The model under review builds one solid part; all positions refer to its coordinate system, in mm. Face numbers are marked on the shaded views. A direction names the side the tool comes from. Give positions to 0.01 mm unless a question says otherwise; leave off trailing zeros. Loops run counter-clockwise (first coordinate to the right, second up) from the corner with the lowest first, then second, coordinate; pieces in that order, holes last. Notation, with made-up numbers: M -29.5,-23.75 L 21.5,-23.75 A21 cw 21.5,4.25 Z; hole C 40.25,-38 d4. An arc over 180 degrees is marked long. Return JSON: item names as keys, results as strings.
```python
from build123d import *

# Parameters (mm, degrees)
BOSS_EXTRUDE1_DEPTH = 3
SKETCH2_R           = 3.8
BOSS_EXTRUDE2_DEPTH = 10
SKETCH3_R           = 1.7
CUT_EXTRUDE1_DEPTH  = 20
SKETCH5_R           = 1.1
SKETCH5_W           = 14
SKETCH5_H           = 24
CUT_EXTRUDE2_DEPTH  = 20
SKETCH6_W           = 3
SKETCH6_H           = 20
BOSS_EXTRUDE3_DEPTH = 50
FILLET2_START       = 7
FILLET2_DEPTH       = 2.5


with BuildPart() as part:
    # Sketch1 → Boss-Extrude1 (new body)
    with BuildSketch(Plane.XY):
        with BuildLine():
            Line((-9.5, 6.480740698), (-9.5, 66.480740698))
            Line((-9.5, 66.480740698), (9.5, 66.480740698))
            Line((9.5, 66.480740698), (9.5, 6.480740698))
            ThreePointArc((9.5, 6.480740698), (0, -11.5), (-9.5, 6.480740698))
        make_face()
    extrude(amount=BOSS_EXTRUDE1_DEPTH)

    # Sketch2 → Boss-Extrude2 (add)
    with BuildSketch(Plane.XY.offset(3)):
        Circle(SKETCH2_R)
    extrude(amount=BOSS_EXTRUDE2_DEPTH)

    # Sketch3 → Cut-Extrude1 (cut)
    with BuildSketch(Plane(origin=(0, 0, 0), x_dir=(-1, 0, 0), z_dir=(0, 0, -1))):
        Circle(SKETCH3_R)
    extrude(amount=-CUT_EXTRUDE1_DEPTH, mode=Mode.SUBTRACT)

    # Sketch5 → Cut-Extrude2 (cut)
    with BuildSketch(Plane(origin=(0, 0, 0), x_dir=(-1, 0, 0), z_dir=(0, 0, -1))):
        with Locations((0, 28.1)):
            Circle(SKETCH5_R)
        with Locations(Location((0, 55.9, 0), (0, 0, 180))):
            Circle(SKETCH5_R)
        with Locations((0, 42)):
            Rectangle(SKETCH5_W, SKETCH5_H)
    extrude(amount=-CUT_EXTRUDE2_DEPTH, mode=Mode.SUBTRACT)

    # Sketch6 → Boss-Extrude3 (add)
    with BuildSketch(Plane(origin=(0, 66.480740698, 0), x_dir=(1, 0, 0), z_dir=(0, 1, 0))):
        with Locations((8, -10)):
            Rectangle(SKETCH6_W, SKETCH6_H)
    extrude(amount=BOSS_EXTRUDE3_DEPTH)

    # Fillet2: read off the stored shape, not the designer's step
    # Fillet2 outline → Fillet2 (add)
    with BuildSketch(Plane.YZ.offset(FILLET2_START)):
        with BuildLine():
            add(Edge.make_bspline(
                [(52.980740698, 3), (66.480740698, 3), (66.480740698, 16.5)],
                knots=[0, 0, 0, 1, 1, 1], degree=2, weights=[1, 0.707106781, 1]))
            Line((52.980740698, 3), (66.480740698, 3))
            Line((66.480740698, 3), (66.480740698, 16.5))
        make_face()
    extrude(amount=FILLET2_DEPTH)


solid = part.part
```
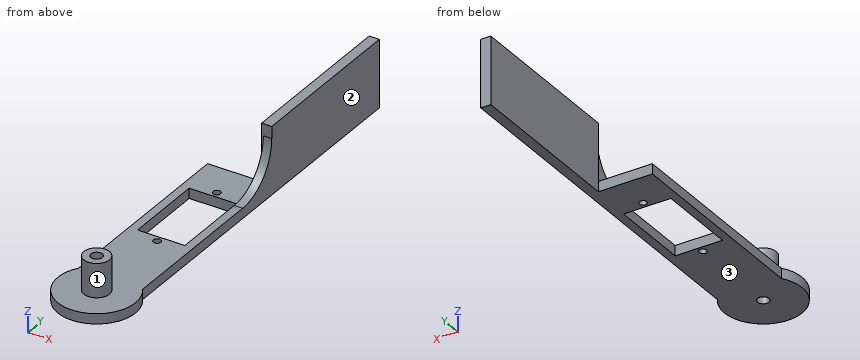
1) Tool access review of the marked faces 1, 2 and 3: name each direction out of +Z, -Z, +X, -X, +Y, -Y from which nothing blocks a thin tool from reaching the whole face with its end or side.
From the geometry:
{"face 1": "+Z", "face 2": "+Z, -Z, +X, +Y", "face 3": "-Z, +X, -X, +Y, -Y"}
2) Consider section C-C on z = 1.5. Write out the cut boundary in (x, y).
From the geometry:
{"outline": "M -9.5,6.48 A11.5 ccw long 9.5,6.48 L 9.5,116.48 L 6.5,116.48 L 6.5,66.48 L -9.5,66.48 Z; hole M -7,30 L 7,30 L 7,54 L -7,54 Z; hole C 0,0 d3.4; hole C 0,28.1 d2.2; hole C 0,55.9 d2.2"}
3) Wall thickness on L1, parallel to Y at x = 0, z = 1.7; L2, parallel to Y at x = 0, z = 7.75; L3, parallel to X at y = 55.9, z = 1.2: over which ranges is each line inside the solid? List them lowest first. Write a range as from..to.
From the geometry:
{"L1": "-11.5..-1.7, 1.7..27, 29.2..30, 54..54.8, 57..66.48", "L2": "-3.8..-1.7, 1.7..3.8", "L3": "-9.5..-1.1, 1.1..9.5"}
4) Consider section D-D on y = 28.1. Write out the cut boundary in (x, z).
From the geometry:
{"outline": "M -9.5,0 L -1.1,0 L -1.1,3 L -9.5,3 Z; M 1.1,0 L 9.5,0 L 9.5,3 L 1.1,3 Z"}
5) Insertion check: pin 1 (0.9 mm diameter, centred on x = -1.5, z = 2, fed in from +Y); pin 2 (1.3 mm diameter, centred on x = 0, y = 55.9, fed in from +Z); pin 3 (12 mm diameter, centred on x = -2.5, z = 15.5, fed in from +Y); pin 4 (0.9 mm diameter, centred on x = 1.5, z = 1.5, fed in from -Y). Each pin has a flat end and moves straight along its axis. Give the tip position at first contact, or say it passes through.
From the geometry:
{"pin 1": "y = 66.48", "pin 2": "through", "pin 3": "y = 3.8", "pin 4": "y = -11.45"}
6) Consider section B-B on y = 0. Write out the cut boundary in (x, z), then the cut area to 3 significant figures.
From the geometry:
{"outline": "M -11.5,0 L -1.7,0 L -1.7,13 L -3.8,13 L -3.8,3 L -11.5,3 Z; M 1.7,0 L 11.5,0 L 11.5,3 L 3.8,3 L 3.8,13 L 1.7,13 Z", "area": "101 mm²"}
7) Consider section A-A on x = 0. Write out the cut boundary in (y, z).
From the geometry:
{"outline": "M -11.5,0 L -1.7,0 L -1.7,13 L -3.8,13 L -3.8,3 L -11.5,3 Z; M 1.7,0 L 27,0 L 27,3 L 3.8,3 L 3.8,13 L 1.7,13 Z; M 29.2,0 L 30,0 L 30,3 L 29.2,3 Z; M 54,0 L 54.8,0 L 54.8,3 L 54,3 Z; M 57,0 L 66.48,0 L 66.48,3 L 57,3 Z"}
